Here's how the part is built. I have some questions about the finished solid (model axes, mm). Round coordinates to 2 decimals unless told otherwise and drop trailing zeros. Write each loop counter-clockwise with the first axis right and the second up, starting at its lowest first coordinate (ties: lowest second). Pieces come first, ordered by that corner, then holes. Notation, with made-up numbers: (32, 9) -> (79, 9) arc R18 cw to (79, 35) -> close; hole circle Ø6 at (58.5, -25). An arc over 180 degrees is marked (long way). Put each result on its own line as item: value. Start each with the question number.
1. Suppose I cut it at A-A (z = 82.99). Please give me the cut outline in (x, y), then the cut area to 3 significant figures.
2. I need wall thicknesses on probe 1 along Z at (x, y) = (5, -60.15); probe 2 along X at (y, z) = (-60.7, 82.99); probe 3 along Y at (x, z) = (0.25, 55). Which ranges of each line are inside material? Lowest first, please. Write a range as from..to.
3. Suppose I cut it at B-B (y = -10). Please give me the cut outline in (x, z).
4. For pin 1 (12 mm diameter, centred on x = -6, y = -6, fed in from -Z); pin 2 (2.5 mm diameter, centred on x = 8, z = 2, fed in from -Y); pin 3 (1.5 mm diameter, centred on x = -1, z = 41, fed in from +Y), each with a flat end and sliding along its axis, tell me the tip position at first contact or that it passes through.
5. Suppose I cut it at C-C (z = 68). Please give me the cut outline in (x, y), then the cut area to 3 significant figures.
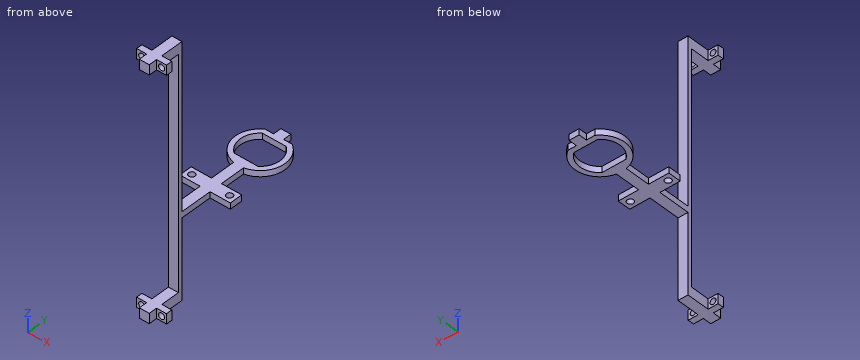
```python
from build123d import *

# Parameters (mm, degrees)
BOSS_EXTRUDE1_DEPTH     = 3
SKETCH3_W               = 25.4
SKETCH3_H               = 6.5
SKETCH3_R               = 1.6
BOSS_EXTRUDE4_DEPTH     = 3
SKETCH11_W              = 5
SKETCH11_H              = 3
BOSS_EXTRUDE8_DEPTH     = 4.15
SKETCH6_W               = 5
SKETCH6_H               = 2
BOSS_EXTRUDE5_DEPTH     = 40
SKETCH10_W              = 5
SKETCH10_H              = 2
BOSS_EXTRUDE7_DEPTH     = 82.49
BOSS_EXTRUDE9_DEPTH     = 5
SKETCH15_R              = 1.5
CUT_EXTRUDE1_DEPTH      = 5
MIRROR2_COPY_1_SKETCH_R = 1.5
MIRROR2_COPY_1_DEPTH    = 5


with BuildPart() as part:
    # Sketch1 → Boss-Extrude1 (new body)
    with BuildSketch(Plane.XY):
        with BuildLine():
            Line((2.5, -49.347448714), (2.5, -12.247448714))
            ThreePointArc((2.5, -12.247448714), (12.284218259, -2.312570382), (6.782329983, 10.5))
            Line((6.782329983, 10.5), (-6.782329983, 10.5))
            ThreePointArc((-6.782329983, 10.5), (-12.284218259, -2.312570382), (-2.5, -12.247448714))
            Line((-2.5, -12.247448714), (-2.5, -49.347448714))
            Line((-2.5, -49.347448714), (2.5, -49.347448714))
        make_face()
        with BuildLine():
            Line((-6, -8), (6, -8))
            ThreePointArc((6, -8), (10, 0), (6, 8))
            Line((6, 8), (-6, 8))
            ThreePointArc((-6, 8), (-10, 0), (-6, -8))
        make_face(mode=Mode.SUBTRACT)
    extrude(amount=BOSS_EXTRUDE1_DEPTH)

    # Sketch3 → Boss-Extrude4 (add)
    with BuildSketch(Plane.XY):
        with Locations((0, -28.097448714)):
            Rectangle(SKETCH3_W, SKETCH3_H)
        with Locations((-9.5, -28.097448714)):
            Circle(SKETCH3_R, mode=Mode.SUBTRACT)
        with Locations(Location((9.5, -28.097448714, 0), (0, 0, 180))):
            Circle(SKETCH3_R, mode=Mode.SUBTRACT)
    extrude(amount=BOSS_EXTRUDE4_DEPTH)

    # Sketch11 → Boss-Extrude8 (add)
    with BuildSketch(Plane(origin=(0, 10.5, 0), x_dir=(1, 0, 0), z_dir=(0, 1, 0))):
        with Locations((0, -1.5)):
            Rectangle(SKETCH11_W, SKETCH11_H)
    extrude(amount=BOSS_EXTRUDE8_DEPTH)

    # Sketch6 → Boss-Extrude5 (add)
    with BuildSketch(Plane(origin=(0, 0, 0), x_dir=(-1, 0, 0), z_dir=(0, 0, -1))):
        with Locations((0, -48.347448714)):
            Rectangle(SKETCH6_W, SKETCH6_H)
    extrude(amount=BOSS_EXTRUDE5_DEPTH)

    # Sketch10 → Boss-Extrude7 (add)
    with BuildSketch(Plane.XY.offset(3)):
        with Locations((0, -48.347448714)):
            Rectangle(SKETCH10_W, SKETCH10_H)
    extrude(amount=BOSS_EXTRUDE7_DEPTH)

    # Sketch14 → Boss-Extrude9 (add)
    with BuildSketch(Plane(origin=(0, 0, -40), x_dir=(-1, 0, 0), z_dir=(0, 0, -1))):
        Polygon((-2.5, -61.767448714), (-2.5, -65.917448714), (2.5, -65.917448714), (2.5, -61.767448714), (7.5, -61.767448714), (7.5, -58.767448714), (2.5, -58.767448714), (2.5, -49.347448714), (-2.5, -49.347448714), (-2.5, -58.767448714), (-7.5, -58.767448714), (-7.5, -61.767448714), align=None)
    boss_extrude9 = extrude(amount=-BOSS_EXTRUDE9_DEPTH)

    # Sketch15 → Cut-Extrude1 (cut)
    with BuildSketch(Plane(origin=(0, -58.767448714, 0), x_dir=(1, 0, 0), z_dir=(0, 1, 0))):
        with Locations(Location((-5, 37.5, 0), (0, 0, 270))):
            Circle(SKETCH15_R)
    cut_extrude1 = extrude(amount=-CUT_EXTRUDE1_DEPTH, mode=Mode.SUBTRACT)

    # Mirror1: Cut-Extrude1 across plane
    add(cut_extrude1.mirror(Plane(origin=(0, 0, 0), x_dir=(0, 0, 1), z_dir=(1, 0, 0))), mode=Mode.SUBTRACT)

    # Mirror2: Boss-Extrude9, Cut-Extrude1 across plane
    add(boss_extrude9.mirror(Plane(origin=(0, 0, 22.745), x_dir=(1, 0, 0), z_dir=(0, 0, -1))))
    add(cut_extrude1.mirror(Plane(origin=(0, 0, 22.745), x_dir=(1, 0, 0), z_dir=(0, 0, -1))), mode=Mode.SUBTRACT)

    # Mirror2 copy 1 sketch → Mirror2 copy 1 (cut)
    with BuildSketch(Plane(origin=(0, -58.767448714, 45.49), x_dir=(-1, 0, 0), z_dir=(0, 1, 0))):
        with Locations(Location((-5, 37.5, 0), (0, 0, 270))):
            Circle(MIRROR2_COPY_1_SKETCH_R)
    extrude(amount=-MIRROR2_COPY_1_DEPTH, mode=Mode.SUBTRACT)


solid = part.part
```
Verdict:
1. outline: (-7.5, -61.77) -> (-6.5, -61.77) -> (-6.5, -58.77) -> (-7.5, -58.77) -> close; (-3.5, -61.77) -> (-2.5, -61.77) -> (-2.5, -65.92) -> (2.5, -65.92) -> (2.5, -61.77) -> (3.5, -61.77) -> (3.5, -58.77) -> (2.5, -58.77) -> (2.5, -47.35) -> (-2.5, -47.35) -> (-2.5, -58.77) -> (-3.5, -58.77) -> close; (6.5, -61.77) -> (7.5, -61.77) -> (7.5, -58.77) -> (6.5, -58.77) -> close
1. area: 105 mm^2
2. probe 1: z = -40..-39, -36..-35, 80.49..81.49, 84.49..85.49
2. probe 2: x = -7.5..-6.5, -3.5..3.5, 6.5..7.5
2. probe 3: y = -49.35..-47.35
3. outline: (-7.5, 0) -> (7.5, 0) -> (7.5, 3) -> (-7.5, 3) -> close
4. pin 1: stops at z = 0
4. pin 2: stops at y = -31.35
4. pin 3: stops at y = -47.35
5. outline: (-2.5, -49.35) -> (2.5, -49.35) -> (2.5, -47.35) -> (-2.5, -47.35) -> close
5. area: 10.0 mm^2
